```python
from build123d import *

# Parameters (mm, degrees)
SKETCH1_R           = 30
BOSS_EXTRUDE1_DEPTH = 35


with BuildPart() as part:
    # Sketch1 → Boss-Extrude1 (new body)
    with BuildSketch(Plane(origin=(0, 0, 0), x_dir=(1, 0, 0), z_dir=(0, 1, 0))):
        with BuildLine():
            Line((-111.539207578, 61.539207578), (-50, 0))
            ThreePointArc((-50, 0), (23.532123251, -44.116200826), (27.849567012, 41.525915008))
            Line((27.849567012, 41.525915008), (-41.425841319, 131.652573837))
            ThreePointArc((-41.425841319, 131.652573837), (-111.539207578, 140.824044377), (-120.710678119, 70.710678119))
            Line((-120.710678119, 70.710678119), (-111.539207578, 61.539207578))
        make_face()
        with Locations(Location((0, 0, 0), (0, 0, 270))):
            Circle(SKETCH1_R, mode=Mode.SUBTRACT)
        with Locations(Location((-81.068259719, 101.181625978, 0), (0, 0, 270))):
            Circle(SKETCH1_R, mode=Mode.SUBTRACT)
    extrude(amount=BOSS_EXTRUDE1_DEPTH)


solid = part.part
```
Build history of the part. All positions in model axes, mm. Give positions to 0.01 mm unless a question says otherwise; leave off trailing zeros. Order: outer loops, then holes, each group sorted by start corner. A loop starts at its lowest first (then second) coordinate and runs counter-clockwise, first axis right, second up. Notation, with made-up numbers: M -16,54.5 L 16,54.5 A8 cw 16,64.5 Z; hole C -28,24.5 d11. An arc over 180 degrees is marked long. Write item = value, one per line. Start each with the question number.
(1) Probe L1, parallel to Z at x = 19, y = 13; L2, parallel to X at y = 25, z = 10.5; L3, parallel to X at y = 7.5, z = -15.5. List the from-to ranges inside material, lowest first. Write a range as [from, to].
(2) Slice it at A-A on z = -89.5. Write the cut outline in (x, y).
(3) Two-plate mould, pull along Z, no slides. Class faces 1 (the flat face through (-6.303, 17.255, -85.958)), 2 (the cylindrical face through (1.32, 17.26, -29.97)), 3 (the cylindrical face through (22.2, 17.3, 44.8)): released by +Z, released by -Z, zero draft, split by the parting line, or undercut.
(4) Slice it at D-D on z = 37.5. Write the cut outline in (x, y), plus the area to 3 significant figures.
(5) Slice it at C-C on y = 19. Write the cut outline in (x, z), plus the area to 3 significant figures.
(6) Pin check, flat tips, straight feed: pin 1 Ø8 at (x, y) = (-9.5, 7) entering from -Z; pin 2 Ø1.5 at (x, y) = (-89, 9) entering from +Z; pin 3 Ø8 at (x, y) = (-103.5, 10) entering from +Z; pin 4 Ø6 at (x, z) = (5.5, -79.5) entering from -Y. Stop position of each tip, or through.
(7) Slice it at B-B on x = 11. Write the cut outline in (y, z) (3 decimals).
Responses:
q1.L1 = [-53.04, -23.22], [23.22, 46.25]
q1.L2 = [-48.89, -28.1], [28.1, 48.89]
q1.L3 = [-65.5, -25.69], [25.69, 47.54]
q2.outline = M -129.68,0 L -108.7,0 L -108.7,35 L -129.68,35 Z; M -53.44,0 L -9.03,0 L -9.03,35 L -53.44,35 Z
q3.face_1 = released by -Z
q3.face_2 = undercut
q3.face_3 = split by the parting line
q4.outline = M -33.07,0 L 33.07,0 L 33.07,35 L -33.07,35 Z
q4.area = 2,320 mm2
q5.outline = M -120.71,-70.71 A50 ccw -41.43,-131.65 L 27.85,-41.53 A50 ccw long -50,0 Z; hole C -81.07,-101.18 d60; hole C 0,0 d60
q5.area = 14,400 mm2
q6.pin_1 = -95.32
q6.pin_2 = -38.25
q6.pin_3 = -49.5
q6.pin_4 = through
q7.outline = M 0,-63.447 L 35,-63.447 L 35,-27.911 L 0,-27.911 Z; M 0,27.911 L 35,27.911 L 35,48.775 L 0,48.775 Z
